Work out the finished part from the listing and answer in its coordinate system (mm). A direction names the side the tool comes from. Round coordinates to 2 decimals unless told otherwise and drop trailing zeros. Order: outer loops, then holes, each group sorted by start corner. A loop starts at its lowest first (then second) coordinate and runs counter-clockwise, first axis right, second up. Notation, with made-up numbers: (-13, 56) - (-4, 56) arc R29 ccw to (-4, 80) - close; hole circle Ø6 at (50, 81). An arc over 180 degrees is marked (long way). One line per question, with ' | ' between items. Start each with the question number.
from build123d import *

# Parameters (mm, degrees)
F0_W     = 6
F0_H     = 13
F0_W_2   = 36
F0_R     = 3
F0_R_2   = 1.5
F1_DEPTH = 0.8
F2_DEPTH = 22
F3_DEPTH = 8.25
F4_R     = 13
F4_W     = 6
F4_H     = 13
F4_R_2   = 9.08
F5_DEPTH = 5.75
F6_R     = 7


# Not quite as in the source:
# - a feature names something its author has since deleted; it is built from what else it names


with BuildPart() as f1:
    # F0 (on Top) → F1 (new body)
    with BuildSketch(Plane.XY):
        with Locations((-3, 6.5)):
            Rectangle(F0_W, F0_H)
        with Locations((-24, 6.5)):
            Rectangle(F0_W_2, F0_H)
        with Locations((-28, 9)):
            Circle(F0_R, mode=Mode.SUBTRACT)
        with Locations((-28, 9)):
            Circle(F0_R)
        with Locations((-28, 9)):
            Circle(F0_R_2, mode=Mode.SUBTRACT)
    extrude(amount=F1_DEPTH)

    # F0 (on Top) → F2 (join)
    with BuildSketch(Plane.XY):
        with Locations((-3, 6.5)):
            Rectangle(F0_W, F0_H)
    extrude(amount=-F2_DEPTH)

    # F0 (on Top) → F3 (join)
    with BuildSketch(Plane.XY):
        with Locations((-24, 6.5)):
            Rectangle(F0_W_2, F0_H)
        with Locations((-28, 9)):
            Circle(F0_R, mode=Mode.SUBTRACT)
    extrude(amount=-F3_DEPTH)

    # F4 (on face) → F5 (join)
    with BuildSketch(Plane(origin=(0, 0, -22), x_dir=(1, 0, 0), z_dir=(0, 0, -1))):
        Polygon((29, 17.66), (-6, 17.66), (-6, 0), (0, 0), (0, -13), (17.6005885005, -13), (29, -13), align=None)
        with Locations((13, 2.33)):
            Circle(F4_R, mode=Mode.SUBTRACT)
        with Locations((-3, -6.5)):
            Rectangle(F4_W, F4_H)
        with Locations((13, 2.33)):
            Circle(F4_R)
        with Locations((13, 2.33)):
            Circle(F4_R_2, mode=Mode.SUBTRACT)
    extrude(amount=F5_DEPTH)

    # F6
    f6_edges = [f1.edges().sort_by_distance(p)[0] for p in [
        (-6, -17.66, -24.875),
        (29, -17.66, -24.875),
        (29, 13, -24.875),
    ]]
    fillet(f6_edges, radius=F6_R)


solid = f1.part
1) Section C-C on z = -2 is taken. Give the vertices of the cut face in (x, y).
2) Straight lines are drawn through the part: line 1 (Y direction, x = 13, z = -23.15); line 2 (Y direction, x = -24.5, z = -5.5); line 3 (Y direction, x = -28, z = -3.75). For each, find the intervals that lie inside material, in ascending order.
3) For faces 1 (the flat face through (-21, 0, -5)), 2 (the cylindrical face through (-31, 9, -4)), 3 (the flat face through (0, 6, -10)), 4 (the flat face through (-6, 4, -20)), determine the directions among +Z, -Z, +X, -X, +Y, -Y from which every point of the face is accessible in a straight line to the end or side of a thin tool.
4) Flat-ended cylindrical pins translate along their axes: pin 1 (10 mm diameter, centred on x = -28.5, y = 5, fed in from -Z); pin 2 (5 mm diameter, centred on y = -1.5, z = -12.5, fed in from +X); pin 3 (2.5 mm diameter, centred on x = -28, y = 9, fed in from +Z); pin 4 (7 mm diameter, centred on x = -26.5, z = -5.5, fed in from -Y). Find the tip coordinate at first contact, or state that the pin passes through.
5) Section D-D on x = 13 is taken. Give the vertices of the cut face in (y, z), and give its area (3 significant figures).
6) Section B-B on y = -8 is taken. Give the vertices of the cut face in (x, z), and give its area (3 significant figures).
7) Section A-A on x = -28 is taken. Give the vertices of the cut face in (y, z), and give its area (4 significant figures).
8) Determine the mould class of faces 5 (the cylindrical face through (27, -15.56, -24.92)), 6 (the cylindrical face through (-29.5, 9.07, 0.39)), 7 (the cylindrical face through (-4, -15.56, -24.92)) for opening direction X: released by +X, released by -X, zero draft, split by the parting line, or undercut.
Recorded:
1) outline: (-42, 0) - (0, 0) - (0, 13) - (-42, 13) - close; hole circle Ø6 at (-28, 9)
2) line 1: y = -17.66 to -11.41, 6.75 to 13 | line 2: y = 0 to 13 | line 3: y = 0 to 6, 12 to 13
3) face 1: +Z, +X, -X, -Y | face 2: -Z | face 3: +Z, +X, +Y, -Y | face 4: -Z, -X, +Y, -Y
4) pin 1: stops at z = -8.25 | pin 2: stops at x = 0 | pin 3: passes through | pin 4: stops at y = 0
5) outline: (-17.66, -27.75) - (-11.41, -27.75) - (-11.41, -22) - (-17.66, -22) - close; (6.75, -27.75) - (13, -27.75) - (13, -22) - (6.75, -22) - close | area: 71.9 mm²
6) outline: (-6, -27.75) - (5.91, -27.75) - (5.91, -22) - (-6, -22) - close; (20.09, -27.75) - (29, -27.75) - (29, -22) - (20.09, -22) - close | area: 120 mm²
7) outline: (0, -8.25) - (6, -8.25) - (6, 0) - (7.5, 0) - (7.5, 0.8) - (0, 0.8) - close; (10.5, 0) - (12, 0) - (12, -8.25) - (13, -8.25) - (13, 0.8) - (10.5, 0.8) - close | area: 65.75 mm²
8) face 5: released by +X | face 6: undercut | face 7: released by -X
